```python
from build123d import *

# Parameters (mm, degrees)
SKETCH1_W           = 300
SKETCH1_H           = 210
BOSS_EXTRUDE1_DEPTH = 5
SKETCH2_W           = 67.619836516
SKETCH2_H           = 30
SKETCH2_W_2         = 72.619836516
SKETCH2_W_3         = 53.212613818
CUT_EXTRUDE1_DEPTH  = 6
SKETCH3_W           = 50
SKETCH3_H           = 110
CUT_EXTRUDE2_DEPTH  = 6


with BuildPart() as part:
    # Sketch1 → Boss-Extrude1 (new body)
    with BuildSketch(Plane.XY):
        Rectangle(SKETCH1_W, SKETCH1_H)
    extrude(amount=BOSS_EXTRUDE1_DEPTH)

    # Sketch2 → Cut-Extrude1 (cut, through all)
    with BuildSketch(Plane(origin=(0, 0, 0), x_dir=(-1, 0, 0), z_dir=(0, 0, -1))):
        with Locations((-178.809918258, 65)):
            Rectangle(SKETCH2_W, SKETCH2_H)
        with Locations((-181.309918258, 5)):
            Rectangle(SKETCH2_W_2, SKETCH2_H)
        with Locations((-181.309918258, -55)):
            Rectangle(SKETCH2_W_2, SKETCH2_H)
        with Locations((171.606306909, 65)):
            Rectangle(SKETCH2_W_3, SKETCH2_H)
        with Locations((181.309918258, 5)):
            Rectangle(SKETCH2_W_2, SKETCH2_H)
        with Locations((181.309918258, -55)):
            Rectangle(SKETCH2_W_2, SKETCH2_H)
    extrude(amount=-CUT_EXTRUDE1_DEPTH, mode=Mode.SUBTRACT)

    # Sketch3 → Cut-Extrude2 (cut, through all)
    with BuildSketch(Plane.XY.offset(5)):
        with Locations((0, -50)):
            Rectangle(SKETCH3_W, SKETCH3_H)
    extrude(amount=-CUT_EXTRUDE2_DEPTH, mode=Mode.SUBTRACT)


solid = part.part
```
The listing builds one solid part. Answer for the finished solid, in the listing's coordinates (mm). Give positions to 0.01 mm unless a question says otherwise; leave off trailing zeros. Order: outer loops, then holes, each group sorted by start corner. A loop starts at its lowest first (then second) coordinate and runs counter-clockwise, first axis right, second up.
Item 1: The part is cut by section C-C, the plane y = 13.5. Give the vertices of the cut face in (x, z).
From the geometry:
outline: (-145, 0) - (145, 0) - (145, 5) - (-145, 5) - close
Item 2: The part is cut by section A-A, the plane y = -59. Give the vertices of the cut face in (x, z).
From the geometry:
outline: (-145, 0) - (-25, 0) - (-25, 5) - (-145, 5) - close; (25, 0) - (145, 0) - (145, 5) - (25, 5) - close
Item 3: Find the intervals of material crossed by probe 1 along X at (y, z) = (-20, 3.35); probe 2 along X at (y, z) = (-58.5, 3.7); probe 3 along Y at (x, z) = (3, 0.65), in increasing order.
From the geometry:
probe 1: x = -150 to -25, 25 to 150
probe 2: x = -145 to -25, 25 to 145
probe 3: y = 5 to 105
